For this review, take the finished solid that the model builds, in its own axes (mm). Coordinates: 2 decimals unless noted, no trailing zeros. Write each loop counter-clockwise with the first axis right and the second up, starting at its lowest first coordinate (ties: lowest second). Pieces come first, ordered by that corner, then holes.
1) To check wall thickness, follow line 1 along Y through (x, z) = (393.5, -3); line 2 along Z through (x, y) = (196, 4); line 3 along Y through (x, z) = (134, -15.5). State the ranges of each line that lie inside material, in increasing order.
2) Insertion check: P1, Ø10, axis at y = -6, z = 24.5, coming from the -X side; P2, Ø12, axis at x = 351.5, y = -21, coming from the +Z side; P3, Ø3, axis at y = -8.5, z = -18.5, coming from the +X side. Each pin has a flat end and moves straight along its axis. Give the tip position at first contact, or say it passes through.
3) We need section B-B on x = 139. Write out the cut boundary in (y, z), then the cut area to 3 significant figures.
4) We need section C-C on y = 12.5. Write out the cut boundary in (x, z), then the cut area to 3 significant figures.
5) We need section A-A on z = 0. Write out the cut boundary in (x, y).
from build123d import *

# Parameters (mm, degrees)
SKETCH1_R           = 31.75
BOSS_EXTRUDE1_DEPTH = 698.5
SKETCH5_R           = 31.75
BOSS_EXTRUDE2_DEPTH = 63.5
SKETCH6_R           = 31.75
BOSS_EXTRUDE3_DEPTH = 63.5
CUT_EXTRUDE1_DEPTH  = 63.5


with BuildPart() as part:
    # Sketch1 → Boss-Extrude1 (new body)
    with BuildSketch(Plane(origin=(0, 0, 0), x_dir=(0, 0, -1), z_dir=(1, 0, 0))):
        Circle(SKETCH1_R)
    extrude(amount=BOSS_EXTRUDE1_DEPTH)

    # Sketch5 → Boss-Extrude2 (add)
    with BuildSketch(Plane.ZY):
        Circle(SKETCH5_R)
    extrude(amount=BOSS_EXTRUDE2_DEPTH)

    # Sketch6 → Boss-Extrude3 (add)
    with BuildSketch(Plane(origin=(698.5, 0, 0), x_dir=(0, 0, -1), z_dir=(1, 0, 0))):
        Circle(SKETCH6_R)
    extrude(amount=BOSS_EXTRUDE3_DEPTH)

    # Sketch7 → Cut-Extrude1 (cut)
    with BuildSketch(Plane(origin=(0, 31.75, 0), x_dir=(1, 0, 0), z_dir=(0, 1, 0))):
        Polygon((0, -31.75), (-63.5, -31.75), (-63.5, 31.75), align=None)
        Polygon((698.5, -31.75), (762, 31.75), (762, -31.75), align=None)
    extrude(amount=-CUT_EXTRUDE1_DEPTH, mode=Mode.SUBTRACT)


solid = part.part
Result:
1. line 1: y = -31.61 to 31.61
1. line 2: z = -31.5 to 31.5
1. line 3: y = -27.71 to 27.71
2. P1: stops at x = -12.25
2. P2: stops at z = 27.98
2. P3: stops at x = 750.25
3. outline: circle Ø63.5 at (0, 0)
3. area: 3,170 mm2
4. outline: (-60.94, -29.19) - (759.44, -29.19) - (701.06, 29.19) - (-2.56, 29.19) - close
4. area: 44,500 mm2
5. outline: (-31.75, -31.75) - (730.25, -31.75) - (730.25, 31.75) - (-31.75, 31.75) - close
